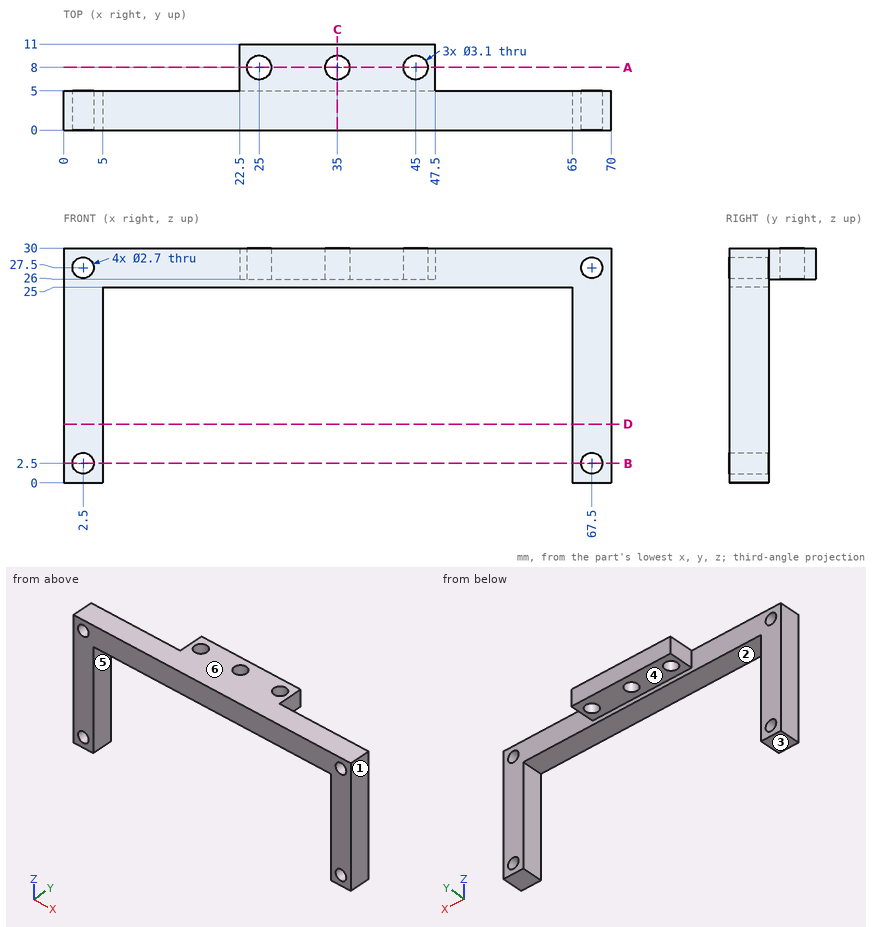
The drawing under review shows one solid part. Ordinate dimensions are in mm from its lowest x, y, z. A direction names the side the tool comes from. Round coordinates to 2 decimals unless told otherwise and drop trailing zeros. Write each loop counter-clockwise with the first axis right and the second up, starting at its lowest first coordinate (ties: lowest second). Pieces come first, ordered by that corner, then holes. Notation, with made-up numbers: (-37, 8.5) - (-20, 8.5) arc R13 ccw to (-20, 12.5) - close; hole circle Ø6 at (84.5, 47.25). An arc over 180 degrees is marked (long way). Write each question's results on one line, items separated by ' | '.
Item 1: For the marked faces 4, 5 and 6, list the 3-axis set-ups (+Z, -Z, +X, -X, +Y, -Y) from which the entire face can be reached by the end or side of a thin tool; tool diameter is ignored.
Calculated:
face 4: -Z, +X, -X, +Y | face 5: -Z, +Y, -Y | face 6: +Z, +X, -X, +Y, -Y
Item 2: For pin 1 (3 mm diameter, centred on y = 9, z = 28.5, fed in from -X); pin 2 (4.5 mm diameter, centred on x = 2.5, z = 27.5, fed in from -Y); pin 3 (3 mm diameter, centred on x = 45, y = 8, fed in from +Z); pin 4 (2.5 mm diameter, centred on x = 49.5, y = 3, fed in from -Z), all flat-tipped, find the tip position at first contact; note any pin that passes through.
Calculated:
pin 1: stops at x = 22.5 | pin 2: stops at y = 0 | pin 3: passes through | pin 4: stops at z = 25
Item 3: Take a section at C-C on x = 35. State the section outline as (y, z) points, then the cut area to 3 significant figures.
Calculated:
outline: (0, 25) - (5, 25) - (5, 26) - (6.45, 26) - (6.45, 30) - (0, 30) - close; (9.55, 26) - (11, 26) - (11, 30) - (9.55, 30) - close | area: 36.6 mm^2
Item 4: Take a section at B-B on z = 2.5. State the section outline as (x, y) points.
Calculated:
outline: (0, 0) - (1.15, 0) - (1.15, 5) - (0, 5) - close; (3.85, 0) - (5, 0) - (5, 5) - (3.85, 5) - close; (65, 0) - (66.15, 0) - (66.15, 5) - (65, 5) - close; (68.85, 0) - (70, 0) - (70, 5) - (68.85, 5) - close
Item 5: Take a section at D-D on z = 7.5. State the section outline as (x, y) points, then the cut area to 3 significant figures.
Calculated:
outline: (0, 0) - (5, 0) - (5, 5) - (0, 5) - close; (65, 0) - (70, 0) - (70, 5) - (65, 5) - close | area: 50.0 mm^2
Item 6: Take a section at A-A on y = 8. State the section outline as (x, z) points, then the cut area to 3 significant figures.
Calculated:
outline: (22.5, 26) - (23.45, 26) - (23.45, 30) - (22.5, 30) - close; (26.55, 26) - (33.45, 26) - (33.45, 30) - (26.55, 30) - close; (36.55, 26) - (43.45, 26) - (43.45, 30) - (36.55, 30) - close; (46.55, 26) - (47.5, 26) - (47.5, 30) - (46.55, 30) - close | area: 62.8 mm^2
Item 7: To check wall thickness, follow line 1 along Z through (x, y) = (67.5, 3.8); line 2 along X through (y, z) = (0.5, 1.5); line 3 along X through (y, z) = (1.75, 18). State the ranges of each line that lie inside material, in increasing order. Write a range as from..to.
Calculated:
line 1: z = 0..1.15, 3.85..26.15, 28.85..30 | line 2: x = 0..1.59, 3.41..5, 65..66.59, 68.41..70 | line 3: x = 0..5, 65..70
Item 8: Draft analysis for pull direction X (two halves, no side actions). For the marked faces 1, 2 and 3, state which applies: pulls with the +X half, pulls with the -X half, needs draft (parallel to the pull), parting line crosses it, or undercut.
Calculated:
face 1: pulls with the +X half | face 2: undercut | face 3: needs draft
